from build123d import *

# Parameters (mm, degrees)
BOSS_EXTRUDE1_DEPTH = 12
SKETCH3_R           = 30
BOSS_EXTRUDE2_DEPTH = 70
SKETCH4_R           = 25
CUT_EXTRUDE1_DEPTH  = 70


with BuildPart() as part:
    # Sketch1 → Boss-Extrude1 (new body)
    with BuildSketch(Plane(origin=(0, 0, 0), x_dir=(1, 0, 0), z_dir=(0, 1, 0))):
        with BuildLine():
            Line((-45, 50), (45, 50))
            ThreePointArc((45, 50), (48.535533906, 48.535533906), (50, 45))
            Line((50, 45), (50, -45))
            ThreePointArc((50, -45), (48.535533906, -48.535533906), (45, -50))
            Line((45, -50), (-45, -50))
            ThreePointArc((-45, -50), (-48.535533906, -48.535533906), (-50, -45))
            Line((-50, -45), (-50, 45))
            ThreePointArc((-50, 45), (-48.535533906, 48.535533906), (-45, 50))
        make_face()
    extrude(amount=BOSS_EXTRUDE1_DEPTH)

    # Sketch3 → Boss-Extrude2 (add)
    with BuildSketch(Plane(origin=(0, 12, 0), x_dir=(1, 0, 0), z_dir=(0, 1, 0))):
        with Locations(Location((0, 0, 0), (0, 0, 270))):
            Circle(SKETCH3_R)
    extrude(amount=BOSS_EXTRUDE2_DEPTH)

    # Sketch4 → Cut-Extrude1 (cut)
    with BuildSketch(Plane(origin=(0, 82, 0), x_dir=(1, 0, 0), z_dir=(0, 1, 0))):
        with Locations(Location((0, 0, 0), (0, 0, 270))):
            Circle(SKETCH4_R)
    extrude(amount=-CUT_EXTRUDE1_DEPTH, mode=Mode.SUBTRACT)


solid = part.part
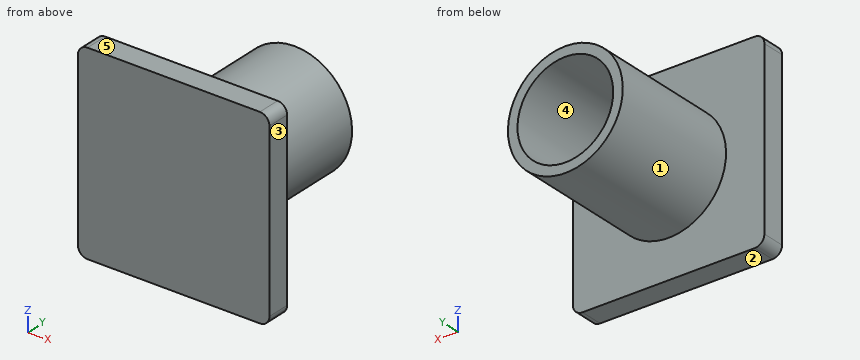
Model file for the job. Use its own axes, mm. Face numbers are marked on the shaded views. A direction names the side the tool comes from. Coordinates: 2 decimals unless noted, no trailing zeros. Order: outer loops, then holes, each group sorted by start corner. A loop starts at its lowest first (then second) coordinate and runs counter-clockwise, first axis right, second up. Notation, with made-up numbers: (9, -39) -> (27, -39) arc R16 cw to (27, -28) -> close; hole circle Ø11 at (-27, 27). An arc over 180 degrees is marked (long way). Return JSON: item names as keys, results as strings. Group by question number.
Item 1: Saw through at B-B on z = 0. Write the cut outline in (x, y), then the cut area to 3 significant figures.
Item 2: Wall check: line 1 along X through (y, z) = (46, 0); line 2 along Y through (x, z) = (12.5, -27.5); line 3 along Z through (x, y) = (19, 68.5). Give the ranges that are in metal, low to high. Write a range as [from, to].
Item 3: Pull direction X, two halves, no side cores. Call the marked faces 3, 4 and 5: pulls with the +X half, pulls with the -X half, needs draft (parallel to the pull), parting line crosses it, or undercut.
Item 4: Saw through at A-A on x = 0. Write the cut outline in (y, z), then the cut area to 3 significant figures.
Item 5: Flat gauge pins, fed straight in: P1, Ø2, axis at y = 41, z = 8.5, coming from the -X side; P2, Ø3, axis at y = 44, z = -1, coming from the -X side; P3, Ø1, axis at x = -5, z = 19.5, coming from the -Y side; P4, Ø5, axis at y = 67, z = -16.5, coming from the -X side. Where does each tip first touch, or does it go through?
Item 6: Saw through at D-D on x = -35.5. Write the cut outline in (y, z), then the cut area to 3 significant figures.
Item 7: Saw through at C-C on y = 41.5. Write the cut outline in (x, z).
Item 8: Tool access for the marked faces 1 and 2: list every direction of +Z, -Z, +X, -X, +Y, -Y with a clear straight run to the whole face (end or side of a thin tool).
Values found:
{
 "1": {"outline": "(-50, 0) -> (50, 0) -> (50, 12) -> (30, 12) -> (30, 82) -> (25, 82) -> (25, 12) -> (-25, 12) -> (-25, 82) -> (-30, 82) -> (-30, 12) -> (-50, 12) -> close", "area": "1,900 mm2"},
 "2": {"line 1": "x = [-30, -25], [25, 30]", "line 2": "y = [0, 12]", "line 3": "z = [-23.22, -16.25], [16.25, 23.22]"},
 "3": {"face 3": "pulls with the +X half", "face 4": "undercut", "face 5": "needs draft"},
 "4": {"outline": "(0, -50) -> (12, -50) -> (12, -30) -> (82, -30) -> (82, -25) -> (12, -25) -> (12, 25) -> (82, 25) -> (82, 30) -> (12, 30) -> (12, 50) -> (0, 50) -> close", "area": "1,900 mm2"},
 "5": {"P1": "stops at x = -29.05", "P2": "stops at x = -30", "P3": "stops at y = 0", "P4": "stops at x = -26.53"},
 "6": {"outline": "(0, -50) -> (12, -50) -> (12, 50) -> (0, 50) -> close", "area": "1,200 mm2"},
 "7": {"outline": "circle Ø60 at (0, 0); hole circle Ø50 at (0, 0)"},
 "8": {"face 1": "+Y", "face 2": "-Z, +X, -X, +Y, -Y"}
}
